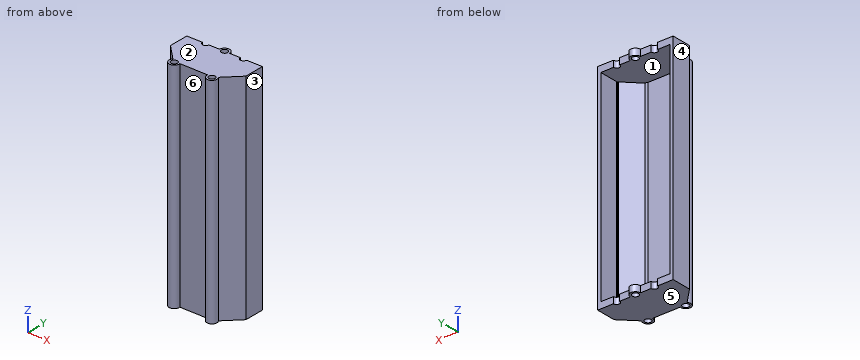
```python
from build123d import *

# Parameters (mm, degrees)
SKETCH1_R               = 6.35
BOSS_EXTRUDE1_DEPTH     = 431.8
CUT_EXTRUDE1_DEPTH      = 12.7
CUT_EXTRUDE1_DEPTH_BACK = 40.64
SKETCH2_W               = 139.7
SKETCH2_H               = 406.4
CUT_EXTRUDE2_START      = -12.7
CUT_EXTRUDE2_DEPTH      = 406.4


with BuildPart() as part:
    # Sketch1 → Boss-Extrude1 (new body)
    with BuildSketch(Plane.XY):
        with BuildLine():
            Line((-61.221298715, -5.681163946), (-61.221298715, 33.973927789))
            Line((-61.221298715, 33.973927789), (-29.471298715, 33.973927789))
            ThreePointArc((-29.471298715, 33.973927789), (-23.121298715, 27.623927789), (-16.771298715, 33.973927789))
            Line((-16.771298715, 33.973927789), (4.818701285, 33.973927789))
            ThreePointArc((4.818701285, 33.973927789), (14.978701285, 44.133927789), (25.138701285, 33.973927789))
            Line((25.138701285, 33.973927789), (46.728701285, 33.973927789))
            ThreePointArc((46.728701285, 33.973927789), (53.078701285, 27.623927789), (59.428701285, 33.973927789))
            Line((59.428701285, 33.973927789), (91.178701285, 33.973927789))
            Line((91.178701285, 33.973927789), (91.178701285, -5.681163946))
            Line((91.178701285, -5.681163946), (60.998251243, -35.861613988))
            ThreePointArc((60.998251243, -35.861613988), (55.706795467, -52.040282366), (43.038417937, -40.670980475))
            Line((43.038417937, -40.670980475), (-13.081015368, -40.670980475))
            ThreePointArc((-13.081015368, -40.670980475), (-25.749392897, -52.040282366), (-31.040848673, -35.861613988))
            Line((-31.040848673, -35.861613988), (-61.221298715, -5.681163946))
        make_face()
        with Locations((14.978701285, 33.973927789)):
            Circle(SKETCH1_R, mode=Mode.SUBTRACT)
        with Locations((53.078701285, -42.226072211)):
            Circle(SKETCH1_R, mode=Mode.SUBTRACT)
        with Locations((-23.121298715, -42.226072211)):
            Circle(SKETCH1_R, mode=Mode.SUBTRACT)
    extrude(amount=BOSS_EXTRUDE1_DEPTH)

    # Sketch2 → Cut-Extrude1 (cut, two sides: drawn at the far end of the back side and taken through both)
    with BuildSketch(Plane(origin=(0, 33.973927789, 0), x_dir=(1, 0, 0), z_dir=(0, 1, 0)).offset(-CUT_EXTRUDE1_DEPTH_BACK)):
        with Locations((14.978701285, -215.9)):
            Rectangle(SKETCH2_W, SKETCH2_H)
    extrude(amount=CUT_EXTRUDE1_DEPTH + CUT_EXTRUDE1_DEPTH_BACK, mode=Mode.SUBTRACT)

    # Sketch3 → Cut-Extrude2 (cut)
    with BuildSketch(Plane(origin=(0, 0, 0), x_dir=(-1, 0, 0), z_dir=(0, 0, -1)).offset(CUT_EXTRUDE2_START)):
        Polygon((-85.778082442, -4.007478335), (56.550022931, -4.007478335), (23.202132139, -37.296656509), (-53.066680528, -37.296656509), align=None)
    extrude(amount=-CUT_EXTRUDE2_DEPTH, mode=Mode.SUBTRACT)


solid = part.part
```
Check sheet for the modelled part. Datum: model origin and axes. Units: mm. Face numbers are marked on the shaded views. A direction names the side the tool comes from. Coordinates: 2 decimals unless noted, no trailing zeros. Order: outer loops, then holes, each group sorted by start corner. A loop starts at its lowest first (then second) coordinate and runs counter-clockwise, first axis right, second up. Notation, with made-up numbers: (50, 43.25) -> (58, 43.25) arc R11 ccw to (58, 52.25) -> close; hole circle Ø1 at (47.25, -39). An arc over 180 degrees is marked (long way). Write each question's results on one line, items separated by ' | '. Start each with the question number.
1) Section check D-D (y = -26.5). Enter the section's corners in (x, z).
2) Section check C-C (x = -8.5). Enter the section's corners in (y, z), and give its area (3 significant figures).
3) Draft check along X on the marked faces 3, 4, 5 and 6. Enter one of: pulls with the +X half, pulls with the -X half, needs draft (parallel to the pull), parting line crosses it, or undercut.
4) Material ranges on line 1 along Z through (x, y) = (54, -24.5); line 2 along X through (y, z) = (-43, 106.5); line 3 along X through (y, z) = (20.5, 297), recorded low to high.
5) Set-up check for the marked faces 1 and 2: record each of +Z, -Z, +X, -X, +Y, -Y from which the full face is reachable in a straight line by a thin tool's end or side.
6) Section check B-B (z = 208.5). Enter the section's corners in (x, y), and give its area (3 significant figures).
7) Section check A-A (y = 23.5). Enter the section's corners in (x, z).
8) Depth check by flat-ended pin: pin 1 (8 mm diameter, centred on x = 43, z = 81.5, fed in from -Y); pin 2 (9.5 mm diameter, centred on x = 76.5, z = 267, fed in from +Y); pin 3 (1.8 mm diameter, centred on x = 84, z = 223, fed in from +Y). Enter the tip coordinate at first touch or a pass-through.
Checked values:
1) outline: (-40.4, 0) -> (70.36, 0) -> (70.36, 431.8) -> (-40.4, 431.8) -> close; hole (-34.02, 12.7) -> (63.68, 12.7) -> (63.68, 419.1) -> (-34.02, 419.1) -> close
2) outline: (-40.67, 0) -> (33.97, 0) -> (33.97, 12.7) -> (-37.3, 12.7) -> (-37.3, 419.1) -> (33.97, 419.1) -> (33.97, 431.8) -> (-40.67, 431.8) -> close | area: 3,270 mm²
3) face 3: pulls with the +X half | face 4: pulls with the -X half | face 5: needs draft | face 6: undercut
4) line 1: 0 to 12.7, 419.1 to 431.8 | line 2: -33.25 to -29.42, -16.82 to -12.99, 42.95 to 46.78, 59.38 to 63.21 | line 3: -61.22 to -54.87, 84.83 to 91.18
5) face 1: +Y | face 2: +Z, +X, -X, +Y, -Y
6) outline: (-61.22, -5.68) -> (-31.04, -35.86) arc R10.16 ccw (long way) to (-13.08, -40.67) -> (43.04, -40.67) arc R10.16 ccw (long way) to (61, -35.86) -> (91.18, -5.68) -> (91.18, 33.97) -> (84.83, 33.97) -> (84.83, -4.01) -> (85.78, -4.01) -> (84.83, -4.97) -> (84.83, -6.67) -> (83.17, -6.67) -> (54.34, -36) arc R6.35 cw (long way) to (49.08, -37.3) -> (-19.12, -37.3) arc R6.35 cw (long way) to (-24.48, -36.02) -> (-53.89, -6.67) -> (-54.87, -6.67) -> (-54.87, -5.68) -> (-56.55, -4.01) -> (-54.87, -4.01) -> (-54.87, 33.97) -> (-61.22, 33.97) -> close | area: 1,380 mm²
7) outline: (-61.22, 0) -> (91.18, 0) -> (91.18, 431.8) -> (-61.22, 431.8) -> close; hole (-54.87, 12.7) -> (84.83, 12.7) -> (84.83, 419.1) -> (-54.87, 419.1) -> close
8) pin 1: y = -50.37 | pin 2: y = -8.62 | pin 3: y = 33.97
